The listing builds one solid part. Answer for the finished solid, in the listing's coordinates (mm). A direction names the side the tool comes from. Give positions to 0.01 mm unless a question says otherwise; leave off trailing zeros. Write each loop counter-clockwise with the first axis right and the second up, starting at its lowest first coordinate (ties: lowest second). Pieces come first, ordered by that corner, then holes.
```python
from build123d import *

# Parameters (mm, degrees)
F1_DEPTH = 65.786
F2_W     = 30.334652
F2_H     = 28.374772
F3_DEPTH = 25.4


with BuildPart() as f1:
    # F0 (on Front) → F1 (new body)
    with BuildSketch(Plane.XZ):
        Polygon((-84.349416, 76.117642), (-114.684075, 76.117642), (-114.684075, -24.425024), (100.258619, -24.425024), (100.258619, 76.117642), (69.923967, 76.117642), (69.923967, 24.977572), (-7.212728, 24.977572), (-84.349416, 24.977572), align=None)
    extrude(amount=-F1_DEPTH)

    # F2 (on face) → F3 (cut)
    with BuildSketch(Plane.XY.offset(76.117642)):
        with Locations((85.091293, 32.893)):
            Rectangle(F2_W, F2_H)
    extrude(amount=-F3_DEPTH, mode=Mode.SUBTRACT)


solid = f1.part
```
Item 1: Consider probe 1 along X at (y, z) = (62, 57); probe 2 along Z at (x, y) = (46, 37); probe 3 along X at (y, z) = (20.5, 65). Determine where each line is inside the solid, lowest interval first.
Conclusion:
probe 1: x = -114.68 to -84.35, 69.92 to 100.26
probe 2: z = -24.43 to 24.98
probe 3: x = -114.68 to -84.35
Item 2: A cutting plane is placed at C-C, the plane x = 15. Give the vertices of the cut face in (y, z), plus the area to 3 significant figures.
Conclusion:
outline: (0, -24.43) - (65.79, -24.43) - (65.79, 24.98) - (0, 24.98) - close
area: 3,250 mm2
Item 3: A cutting plane is placed at D-D, the plane y = 60. Give the vertices of the cut face in (x, z), plus the area to 3 significant figures.
Conclusion:
outline: (-114.68, -24.43) - (100.26, -24.43) - (100.26, 76.12) - (69.92, 76.12) - (69.92, 24.98) - (-84.35, 24.98) - (-84.35, 76.12) - (-114.68, 76.12) - close
area: 13,700 mm2
Item 4: A cutting plane is placed at B-B, the plane y = 31.5. Give the vertices of the cut face in (x, z), plus the area to 3 significant figures.
Conclusion:
outline: (-114.68, -24.43) - (100.26, -24.43) - (100.26, 50.72) - (69.92, 50.72) - (69.92, 24.98) - (-84.35, 24.98) - (-84.35, 76.12) - (-114.68, 76.12) - close
area: 13,000 mm2
Item 5: A cutting plane is placed at A-A, the plane z = 36.5. Give the vertices of the cut face in (x, y).
Conclusion:
outline: (-114.68, 0) - (-84.35, 0) - (-84.35, 65.79) - (-114.68, 65.79) - close; (69.92, 0) - (100.26, 0) - (100.26, 65.79) - (69.92, 65.79) - close
Item 6: Each of these flat-tipped pins is pushed along its axis until it touches: P1, Ø12, axis at y = 32, z = 51.5, coming from the +X side; P2, Ø8, axis at x = 14, y = 18, coming from the +Z side. Where does it stop, or does it pass through?
Conclusion:
P1: stops at x = 100.26
P2: stops at z = 24.98
Item 7: Which of the six approach directions +Z, -Z, +X, -X, +Y, -Y give full straight-line access (tool end or side, diameter ignored) to faces 4 (the face through (-6, 32, 24.978)), 5 (the face through (85, 56, 76.118)), 6 (the face through (85, 18.706, 64))?
Conclusion:
face 4: +Z, +Y, -Y
face 5: +Z, +X, -X, +Y, -Y
face 6: +Z, +X
Item 8: Determine the mould class of faces 1 (the face through (85, 33, 50.718)), 2 (the face through (100.259, 32, 25)), 3 (the face through (-84.349, 32, 50)) for opening direction X: pulls with the +X half, pulls with the -X half, needs draft (parallel to the pull), parting line crosses it, or undercut.
Conclusion:
face 1: needs draft
face 2: pulls with the +X half
face 3: undercut
